```python
from build123d import *

# Parameters (mm, degrees)
SKETCH1_R           = 48
BOSS_EXTRUDE1_DEPTH = 10
FILLET1_R           = 40


with BuildPart() as part:
    # Sketch1 → Boss-Extrude1 (new body)
    with BuildSketch(Plane(origin=(0, 0, 0), x_dir=(1, 0, 0), z_dir=(0, 1, 0))):
        with BuildLine():
            Line((35, 78), (-35, 78))
            Line((-35, 78), (-35, 48))
            add(Edge.make_bspline(
                [(-35, 48), (-34.99357519, 42.516288621), (-42.093715926, 32.204333242)],
                knots=[0, 0, 0, 1, 1, 1], degree=2))
            ThreePointArc((-42.093715926, 32.204333242), (0, -53), (42.093715926, 32.204333242))
            add(Edge.make_bspline(
                [(35, 48), (34.99357519, 42.516288621), (42.093715926, 32.204333242)],
                knots=[0, 0, 0, 1, 1, 1], degree=2))
            Line((35, 48), (35, 78))
        make_face()
        with Locations(Location((0, 0, 0), (0, 0, 270))):
            Circle(SKETCH1_R, mode=Mode.SUBTRACT)
    extrude(amount=BOSS_EXTRUDE1_DEPTH)

    # Fillet1
    # the kernel refuses this fillet: 40 mm, written as the material it takes off along each edge
    with BuildSketch(Plane(origin=(101.143782777, 10, -78), x_dir=(0, -1, 0), z_dir=(-1, 0, 0))) as fillet1_piece_1:
        with BuildLine():
            CenterArc((40, 26.457513111), FILLET1_R, 180, 41.409622109)
            Line((0, 26.457513111), (-0.8, 26.457513111))
            Line((-0.8, 26.457513111), (-0.8, 0))
            Line((-0.8, 0), (0, -0.8))
            ThreePointArc((0, -0.8), (5, -0.8), (9.4, -0.529150262))
            Line((9.4, -0.529150262), (10, 0))
        make_face()
    extrude(amount=202.287565553, mode=Mode.SUBTRACT)


solid = part.part
```
For this review, take the finished solid that the model builds, in its own axes (mm). A direction names the side the tool comes from. Round coordinates to 2 decimals unless told otherwise and drop trailing zeros. Write each loop counter-clockwise with the first axis right and the second up, starting at its lowest first coordinate (ties: lowest second). Pieces come first, ordered by that corner, then holes. Notation, with made-up numbers: (-17.5, -29.5) - (8.5, -29.5) arc R20 cw to (8.5, -4.5) - close; hole circle Ø6 at (41, 55). An arc over 180 degrees is marked (long way). Answer as a JSON object with one key per item and string values.
1. For pin 1 Ø1 at (y, z) = (6, -2) entering from +X; pin 2 Ø2 at (x, y) = (-31.5, 5.5) entering from -Z; pin 3 Ø1 at (y, z) = (7, -40) entering from -X, all flat-tipped, find the tip position at first contact; note any pin that passes through.
Response values:
{"pin 1": "stops at x = 52.98", "pin 2": "stops at z = -71.78", "pin 3": "stops at x = -37.64"}
2. We need section B-B on z = 0. Give the boundary of the cut face in (x, y), then the cut area to 3 significant figures.
Response values:
{"outline": "(-53, 0) - (-48, 0) - (-48, 10) - (-53, 10) - close; (48, 0) - (53, 0) - (53, 10) - (48, 10) - close", "area": "100 mm2"}
3. Draft analysis for pull direction X (two halves, no side actions). For faces 3 (the face through (-35, 4, -60)), 4 (the face through (15, 10, -46)), 5 (the face through (14.418, 4.93, 45.783)), state which applies: +X half, -X half, draft (parallel to the pull), parting line (faces both ways), or undercut.
Response values:
{"face 3": "-X half", "face 4": "draft", "face 5": "undercut"}
4. Tool access review of faces 1 (the face through (-4, 0, -52)), 2 (the face through (35, 4, -59)): name each direction out of +Z, -Z, +X, -X, +Y, -Y from which nothing blocks a thin tool from reaching the whole face with its end or side.
Response values:
{"face 1": "+Z, -Z, +X, -X, -Y", "face 2": "-Z, +X, +Y, -Y"}
5. To check wall thickness, follow line 1 along X through (y, z) = (2.75, 0); line 2 along Z through (x, y) = (27.5, 7); line 3 along Z through (x, y) = (-17, 2). State the ranges of each line that lie inside material, in increasing order.
Response values:
{"line 1": "x = -53 to -48, 48 to 53", "line 2": "z = -66.74 to -39.34, 39.34 to 45.31", "line 3": "z = -75.54 to -44.89, 44.89 to 50.2"}
6. We need section A-A on x = 0. Give the boundary of the cut face in (y, z), then the cut area to 3 significant figures.
Response values:
{"outline": "(0, -78) arc R40 ccw to (10, -51.54) - (10, -48) - (0, -48) - close; (0, 48) - (10, 48) - (10, 53) - (0, 53) - close", "area": "267 mm2"}
